```python
from build123d import *

# Parameters (mm, degrees)
BOSS_EXTRUDE1_DEPTH     = 3.5
CUT_EXTRUDE1_DEPTH      = 7.975373347
CUT_EXTRUDE1_DEPTH_BACK = 7.975373347
SKETCH2_R               = 2.5
SKETCH4_OUTSIDE_W       = 79.412
SKETCH4_OUTSIDE_H       = 80.634
SKETCH4_OUTSIDE_R       = 3.95
CUT_EXTRUDE4_DEPTH      = 33.5
CUT_EXTRUDE4_DRAFT      = -45


# Read off the part's stored shape, not the designer's step: Cut-Extrude2
with BuildPart() as part:
    # Sketch1 → Boss-Extrude1 (new body)
    with BuildSketch(Plane(origin=(0, 0, 0), x_dir=(1, 0, 0), z_dir=(0, 1, 0))):
        Polygon((3.95, -2.280533563), (3.95, 2.280533563), (0, 4.561067127), (-3.95, 2.280533563), (-3.95, -2.280533563), (0, -4.561067127), align=None)
    extrude(amount=BOSS_EXTRUDE1_DEPTH)

    # Sketch2 → Cut-Extrude1 (cut, two sides: drawn at the far end of the back side and taken through both)
    with BuildSketch(Plane(origin=(0, 3.5, 0), x_dir=(1, 0, 0), z_dir=(0, 1, 0)).offset(-CUT_EXTRUDE1_DEPTH_BACK)):
        with Locations(Location((0, 0, 0), (0, 0, 270))):
            Circle(SKETCH2_R)
    extrude(amount=CUT_EXTRUDE1_DEPTH + CUT_EXTRUDE1_DEPTH_BACK, mode=Mode.SUBTRACT)

    # Cut-Extrude2 outline → Cut-Extrude2 (revolve, cut)
    with BuildSketch(Plane.XY):
        Polygon((4.561067183, 3.500000074), (3.949999968, 3.500000074), (4.561067135, 2.888932865), align=None)
    revolve(axis=Axis((0, 0, 0), (0, 1, 0)), mode=Mode.SUBTRACT)


with BuildPart() as cut_extrude4_tool:
    # Sketch4 outside → Cut-Extrude4 (with draft: the straight prism first)
    with BuildSketch(Plane.XZ):
        Rectangle(SKETCH4_OUTSIDE_W, SKETCH4_OUTSIDE_H)
        Circle(SKETCH4_OUTSIDE_R, mode=Mode.SUBTRACT)
    extrude(amount=-CUT_EXTRUDE4_DEPTH)
    # Cut-Extrude4: the draft: its side faces are tilted about the plane it starts from
    cut_extrude4_sides = [cut_extrude4_tool.faces().sort_by_distance(p)[0] for p in [
        (0, 16.75, -40.317),
        (39.706, 16.75, 0),
        (0, 16.75, 40.317),
        (-39.706, 16.75, 0),
        (-3.95, 16.75, 0),
    ]]
    draft(cut_extrude4_sides, Plane.XZ, CUT_EXTRUDE4_DRAFT)


with BuildPart() as part_1:
    add(part.part)

    # Cut-Extrude4: cut by cut_extrude4_tool
    add(cut_extrude4_tool.part, mode=Mode.SUBTRACT)


solid = part_1.part
```
Verification items for the finished model (mm, model axes). Coordinates: 2 decimals unless noted, no trailing zeros. Write each loop counter-clockwise with the first axis right and the second up, starting at its lowest first coordinate (ties: lowest second). Pieces come first, ordered by that corner, then holes. Notation, with made-up numbers: M 19,42 L 61,42 A30 cw 61,72 Z; hole C 78,65.5 d3. An arc over 180 degrees is marked long. One line per item, written item: value.
Item 1: Scan lines: line 1 along X through (y, z) = (0.5, 0); line 2 along X through (y, z) = (1.75, -1.25); line 3 along Z through (x, y) = (1.25, 1.6). Record each from-to range of solid material in increasing order.
Check sheet entries:
line 1: x = -3.95 to -2.5, 2.5 to 3.95
line 2: x = -3.95 to -2.17, 2.17 to 3.95
line 3: z = -3.84 to -2.17, 2.17 to 3.84
Item 2: Section check A-A, the plane y = 2.7. Record the boundary of the cut face in (x, z), plus the area to 3 significant figures.
Check sheet entries:
outline: M -3.95,-2.28 L 0,-4.56 L 3.95,-2.28 L 3.95,2.28 L 0,4.56 L -3.95,2.28 Z; hole C 0,0 d5
area: 34.4 mm^2
Item 3: Mould release check, pull along Z, two halves, no side actions. Record for faces 1 (the conical face through (3.542, 0.146, -2.057)), 2 (the cylindrical face through (-2.44, 1.73, -0.54)), 3 (the conical face through (3.544, 3.351, 2.058)), 4 (the flat face through (0, 0, 3)): pulls with the +Z half, pulls with the -Z half, needs draft (parallel to the pull), parting line crosses it, or undercut.
Check sheet entries:
face 1: pulls with the -Z half
face 2: undercut
face 3: pulls with the +Z half
face 4: needs draft
